CAD build for the part. Positions are in the model's coordinates, mm. A direction names the side the tool comes from. Round coordinates to 2 decimals unless told otherwise and drop trailing zeros. Write each loop counter-clockwise with the first axis right and the second up, starting at its lowest first coordinate (ties: lowest second). Pieces come first, ordered by that corner, then holes. Notation, with made-up numbers: (28.5, -33) -> (63.5, -33) arc R17 ccw to (63.5, -6) -> close; hole circle Ø2 at (66, -1.5). An arc over 180 degrees is marked (long way). Answer in a Markdown table with one row per item. Add a question column.
Autodesk Inventor part; units mm, degrees
ref_plane "YZ Plane" through (0, 0, 0) normal (1, 0, 0) x (0, 1, 0)
ref_plane "XZ Plane" through (0, 0, 0) normal (0, 1, 0) x (-1, 0, 0)
ref_plane "XY Plane" through (0, 0, 0) normal (0, 0, 1) x (1, 0, 0)
sketch "Sketch1" plane through (0, 0, 0) normal (0, 0, 1) x (1, 0, 0)
  line L0 (5, -6) -> (-5, -6)
  circle A0 centre (0, 31.25) radius 1.5
  arc A1 (5, 31.25) -> (-5, 31.25) centre (0, 31.25) ccw
  line L1 (-5, -6) -> (-5, 31.25)
  line L2 (5, -6) -> (5, 31.25)
  point P0 (0, 0)
  point P1 (0, 0)
  point P2 (0, -6)
  point P3 (0, -6)
  dimension "d2" = 3
  dimension "d13" = 10
  dimension "d15" = 37.25
  dimension "d16" = 6
extrude "Extrusion1" add sketch "Sketch1" along normal blind 3
sketch "Sketch2" plane through (0, 0, 3) normal (0, 0, 1) x (1, 0, 0)
  line L0 (10, -6) -> (10, -9)
  line L1 (10, -9) -> (-10, -9)
  line L2 (-5, -6) -> (5, -6)
  line L3 (5, -6) -> (5, 31.25)
  line L4 (10, -6) -> (-10, -6)
  line L5 (-10, -6) -> (-10, -9)
  line L6 (-5, 31.25) -> (-5, -6)
  point P0 (0, 0)
  dimension "d5" = 3
  dimension "d17" = 5
  dimension "d18" = 5
extrude "Extrusion2" add sketch "Sketch2" against normal blind 3
fillet "Fillet1" radius 1 2 edges at (-10, -9, 1.5) (10, -9, 1.5)
properties part number "arm3"
Item 1: Two-plate mould, pull along Y, no slides. Class faces 4 (the cylindrical face through (-0.11, 36.25, 1.48)), 5 (the cylindrical face through (-0.195, 29.763, 1.479)), 6 (the flat face through (0, 9, 0)): +Y half, -Y half, draft (parallel to the pull), parting line (faces both ways), or undercut.
Item 2: Pin check, flat tips, straight feed: pin 1 (1 mm diameter, centred on y = -2.5, z = 1.5, fed in from -X); pin 2 (1.5 mm diameter, centred on x = 7.5, z = 2, fed in from +Y); pin 3 (1.5 mm diameter, centred on y = 21, z = 1, fed in from +X); pin 4 (3.5 mm diameter, centred on x = 0, y = 31.25, fed in from -Z). Stop position of each tip, or through.
Item 3: Saw through at D-D on x = -6.25. Give the cut face in (y, z), then the cut area to 3 significant figures.
Item 4: Tool access for faces 1 (the flat face through (0, -9, 2)), 2 (the flat face through (5, 12, 1)), 3 (the flat face through (-5, 12, 1)): list every direction of +Z, -Z, +X, -X, +Y, -Y with a clear straight run to the whole face (end or side of a thin tool).
Item 5: Drill centre lines: probe 1 along Y at (x, z) = (0, 1.8); probe 2 along X at (y, z) = (-2, 0.4); probe 3 along Y at (x, z) = (5.75, 2.55). Where is each one in solid material? Low to high.
Item 6: Saw through at A-A on x = 0. Give the cut face in (y, z), then the cut area to 3 significant figures.
Item 7: Saw through at B-B on z = 1.15. Give the cut face in (x, y).
Item 8: Saw through at C-C on y = 29. Give the cut face in (x, z).
Recorded:
| question | item | result |
|---|---|---|
| 1 | face 4 | +Y half |
| 1 | face 5 | undercut |
| 1 | face 6 | draft |
| 2 | pin 1 | x = -5 |
| 2 | pin 2 | y = -6 |
| 2 | pin 3 | x = 5 |
| 2 | pin 4 | z = 0 |
| 3 | outline | (-9, 0) -> (-6, 0) -> (-6, 3) -> (-9, 3) -> close |
| 3 | area | 9.00 mm2 |
| 4 | face 1 | +Z, -Z, +X, -X, -Y |
| 4 | face 2 | +Z, -Z, +X, +Y |
| 4 | face 3 | +Z, -Z, -X, +Y |
| 5 | probe 1 | -9 to 29.75, 32.75 to 36.25 |
| 5 | probe 2 | -5 to 5 |
| 5 | probe 3 | -9 to -6 |
| 6 | outline | (-9, 0) -> (29.75, 0) -> (29.75, 3) -> (-9, 3) -> close; (32.75, 0) -> (36.25, 0) -> (36.25, 3) -> (32.75, 3) -> close |
| 6 | area | 127 mm2 |
| 7 | outline | (-10, -8) arc R1 ccw to (-9, -9) -> (9, -9) arc R1 ccw to (10, -8) -> (10, -6) -> (5, -6) -> (5, 31.25) arc R5 ccw to (-5, 31.25) -> (-5, -6) -> (-10, -6) -> close; hole circle Ø3 at (0, 31.25) |
| 8 | outline | (-5, 0) -> (5, 0) -> (5, 3) -> (-5, 3) -> close |
